from build123d import *

# Parameters (mm, degrees)
SKETCH_W        = 50
SKETCH_H        = 60
PAD_DEPTH       = 4
SKETCH001_W     = 26
SKETCH001_H     = 26
POCKET_DEPTH    = 5
SKETCH003_W     = 50
SKETCH003_H     = 17
PAD001_DEPTH    = 10
SKETCH004_W     = 12
SKETCH004_H     = 43
PAD002_DEPTH    = 10
SKETCH005_W     = 12
SKETCH005_H     = 43
PAD003_DEPTH    = 10
SKETCH006_W     = 50
SKETCH006_H     = 5
POCKET001_DEPTH = 5
SKETCH007_W     = 50
SKETCH007_H     = 5
POCKET002_DEPTH = 5
SKETCH008_W     = 26
SKETCH008_H     = 5
POCKET003_DEPTH = 7
SKETCH009_R     = 2
POCKET004_DEPTH = 15
SKETCH010_R     = 2
POCKET005_DEPTH = 15
SKETCH011_R     = 2
POCKET006_DEPTH = 15
SKETCH014_W     = 26
SKETCH014_H     = 17
POCKET008_DEPTH = 5
SKETCH015_W     = 50
SKETCH015_H     = 60
PAD005_DEPTH    = 3.1445
POCKET009_DEPTH = 50
SKETCH018_W     = 26
SKETCH018_H     = 43
POCKET010_DEPTH = 5
SKETCH019_W     = 50
SKETCH019_H     = 17.1445
PAD006_DEPTH    = 24
SKETCH020_R     = 3.4
POCKET011_DEPTH = 24
SKETCH021_R     = 3.4
POCKET012_DEPTH = 24


with BuildPart() as part:
    # Sketch → Pad (new body)
    with BuildSketch(Plane.XY):
        with Locations((-25, -30)):
            Rectangle(SKETCH_W, SKETCH_H)
    extrude(amount=PAD_DEPTH)

    # Sketch001 → Pocket (cut)
    with BuildSketch(Plane.XY.offset(4)):
        with Locations((-25, -30)):
            Rectangle(SKETCH001_W, SKETCH001_H)
    extrude(amount=-POCKET_DEPTH, mode=Mode.SUBTRACT)

    # Sketch003 → Pad001 (new body)
    with BuildSketch(Plane.XY.offset(4)):
        with Locations((-25, -51.5)):
            Rectangle(SKETCH003_W, SKETCH003_H)
    extrude(amount=PAD001_DEPTH)

    # Sketch004 → Pad002 (new body)
    with BuildSketch(Plane.XY.offset(4)):
        with Locations((-44, -21.5)):
            Rectangle(SKETCH004_W, SKETCH004_H)
    extrude(amount=PAD002_DEPTH)

    # Sketch005 → Pad003 (new body)
    with BuildSketch(Plane.XY.offset(4)):
        with Locations((-6, -21.5)):
            Rectangle(SKETCH005_W, SKETCH005_H)
    extrude(amount=PAD003_DEPTH)

    # Sketch006 → Pocket001 (cut)
    with BuildSketch(Plane.YZ.offset(-38)):
        with Locations((-25, 6.5)):
            Rectangle(SKETCH006_W, SKETCH006_H)
    extrude(amount=-POCKET001_DEPTH, mode=Mode.SUBTRACT)

    # Sketch007 → Pocket002 (cut)
    with BuildSketch(Plane(origin=(-12, 0, 0), x_dir=(0, -1, 0), z_dir=(-1, 0, 0))):
        with Locations((25, 6.5)):
            Rectangle(SKETCH007_W, SKETCH007_H)
    extrude(amount=-POCKET002_DEPTH, mode=Mode.SUBTRACT)

    # Sketch008 → Pocket003 (cut)
    with BuildSketch(Plane(origin=(0, -43, 0), x_dir=(-1, 0, 0), z_dir=(0, 1, 0))):
        with Locations((25, 6.5)):
            Rectangle(SKETCH008_W, SKETCH008_H)
    extrude(amount=-POCKET003_DEPTH, mode=Mode.SUBTRACT)

    # Sketch009 → Pocket004 (cut)
    with BuildSketch(Plane.XY.offset(14)):
        with Locations((-25, -54)):
            Circle(SKETCH009_R)
    extrude(amount=-POCKET004_DEPTH, mode=Mode.SUBTRACT)

    # Sketch010 → Pocket005 (cut)
    with BuildSketch(Plane.XY.offset(14)):
        with Locations((-46.5, -4)):
            Circle(SKETCH010_R)
    extrude(amount=-POCKET005_DEPTH, mode=Mode.SUBTRACT)

    # Sketch011 → Pocket006 (cut)
    with BuildSketch(Plane.XY.offset(14)):
        with Locations((-3.5, -4)):
            Circle(SKETCH011_R)
    extrude(amount=-POCKET006_DEPTH, mode=Mode.SUBTRACT)

    # Sketch014 → Pocket008 (cut)
    with BuildSketch(Plane.XY.offset(4)):
        with Locations((-25, -8.5)):
            Rectangle(SKETCH014_W, SKETCH014_H)
    extrude(amount=-POCKET008_DEPTH, mode=Mode.SUBTRACT)

    # Sketch015 → Pad005 (new body)
    with BuildSketch(Plane(origin=(0, 0, 0), x_dir=(1, 0, 0), z_dir=(0, 0, -1))):
        with Locations((-25, 30)):
            Rectangle(SKETCH015_W, SKETCH015_H)
    extrude(amount=PAD005_DEPTH)

    # Sketch017 → Pocket009 (cut)
    with BuildSketch(Plane(origin=(-50, 0, 0), x_dir=(0, -1, 0), z_dir=(-1, 0, 0))):
        Polygon((0, 0), (0, -3.1445), (60, -3.1445), align=None)
    extrude(amount=-POCKET009_DEPTH, mode=Mode.SUBTRACT)

    # Sketch018 → Pocket010 (cut)
    with BuildSketch(Plane.XY):
        with Locations((-25, -21.5)):
            Rectangle(SKETCH018_W, SKETCH018_H)
    extrude(amount=-POCKET010_DEPTH, mode=Mode.SUBTRACT)

    # Sketch019 → Pad006 (new body)
    with BuildSketch(Plane.XZ.offset(60)):
        with Locations((-25, 5.42775)):
            Rectangle(SKETCH019_W, SKETCH019_H)
    extrude(amount=PAD006_DEPTH)

    # Sketch020 → Pocket011 (cut)
    with BuildSketch(Plane.XZ.offset(84)):
        with Locations((-37.5, 5.4277)):
            Circle(SKETCH020_R)
    extrude(amount=-POCKET011_DEPTH, mode=Mode.SUBTRACT)

    # Sketch021 → Pocket012 (cut)
    with BuildSketch(Plane.XZ.offset(84)):
        with Locations((-12.5, 5.4277)):
            Circle(SKETCH021_R)
    extrude(amount=-POCKET012_DEPTH, mode=Mode.SUBTRACT)


solid = part.part
CAD build for the part. Positions are in the model's coordinates, mm. A direction names the side the tool comes from. Round coordinates to 2 decimals unless told otherwise and drop trailing zeros. Loops run counter-clockwise (first coordinate to the right, second up) from the corner with the lowest first, then second, coordinate; pieces in that order, holes last.
(1) Cut at A-A (y = -4). Give the cut face in (x, z).
(2) Cut at B-B (x = -25). Give the cut face in (y, z), plus the area to 3 significant figures.
(3) Cut at C-C (z = 12.5). Give the cut face in (x, y).
(4) Two-plate mould, pull along X, no slides. Class faces 6 (the flat face through (-23.8, -43.4, 9)), 7 (the flat face through (-44, 0, 7)), 8 (the flat face through (-25, -54, 0)): +X half, -X half, draft (parallel to the pull), parting line (faces both ways), or undercut.
(5) Cut at D-D (y = -38). Give the cut face in (x, z).
(6) Wall check: line 1 along Y through (x, z) = (-3.5, 3); line 2 along Y through (x, z) = (-25, 8.5); line 3 along X through (y, z) = (-40.5, 13.25). Give the ranges that are in metal, low to high.
(7) Which spindle directions (+Z, -Z, +X, -X, +Y, -Y) get a long thin tool onto all of the face, cutting with end or side? Do faces 1 (the flat face through (-38, -22, 11)), 2 (the flat face through (-25, -50, 6)), 3 (the flat face through (-4, -4, 0)), 4 (the cylindrical face through (-13.2, -72.2, 2.1)), 5 (the flat face through (-25, -51, 14)). Say none if no direction does.
(8) Drop flat-ended pins along their axis: pin 1 (2.5 mm diameter, centred on x = -25, y = -54, fed in from +Z); pin 2 (10 mm diameter, centred on x = -35.5, y = -33, fed in from -Z); pin 3 (5.5 mm diameter, centred on x = -23, z = 11, fed in from +Y). Give the stop position or say it passes through.
Findings below:
1. outline: (-50, -0.21) - (-38, -0.21) - (-38, 4) - (-43, 4) - (-43, 9) - (-38, 9) - (-38, 14) - (-44.5, 14) - (-44.5, 0) - (-48.5, 0) - (-48.5, 14) - (-50, 14) - close; (-12, -0.21) - (0, -0.21) - (0, 14) - (-1.5, 14) - (-1.5, 0) - (-5.5, 0) - (-5.5, 14) - (-12, 14) - (-12, 9) - (-7, 9) - (-7, 4) - (-12, 4) - close
2. outline: (-84, -3.14) - (-60, -3.14) - (-43, -2.25) - (-43, 4) - (-50, 4) - (-50, 9) - (-43, 9) - (-43, 14) - (-52, 14) - (-52, 0) - (-56, 0) - (-56, 14) - (-84, 14) - close
2. area: 604 mm2
3. outline: (-50, -84) - (0, -84) - (0, 0) - (-12, 0) - (-12, -43) - (-38, -43) - (-38, 0) - (-50, 0) - close; hole circle Ø4 at (-46.5, -4); hole circle Ø4 at (-25, -54); hole circle Ø4 at (-3.5, -4)
4. face 6: undercut
4. face 7: draft
4. face 8: undercut
5. outline: (-50, -1.99) - (-38, -1.99) - (-38, 4) - (-43, 4) - (-43, 9) - (-38, 9) - (-38, 14) - (-50, 14) - close; (-12, -1.99) - (0, -1.99) - (0, 14) - (-12, 14) - (-12, 9) - (-7, 9) - (-7, 4) - (-12, 4) - close
6. line 1: y = -84 to -6, -2 to 0
6. line 2: y = -84 to -56, -52 to -50
6. line 3: x = -50 to -38, -12 to 0
7. face 1: +Z, -Z, +Y
7. face 2: +Y
7. face 3: +Z
7. face 4: -Y
7. face 5: +Z, +X, -X, +Y, -Y
8. pin 1: stops at z = 0
8. pin 2: stops at z = -1.96
8. pin 3: stops at y = -43
